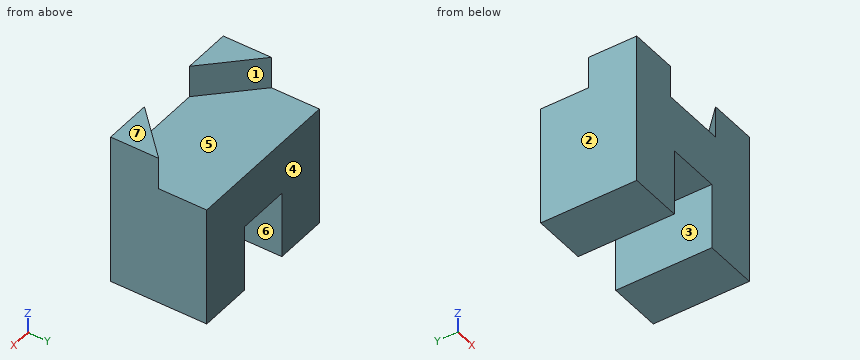
from build123d import *

# Parameters (mm, degrees)
F0_W     = 600
F0_H     = 360
F1_DEPTH = 450
F2_W     = 200
F2_H     = 250
F3_DEPTH = 360.001
F5_DEPTH = 120


with BuildPart() as f1:
    # F0 (on Top) → F1 (new body)
    with BuildSketch(Plane.XY):
        Rectangle(F0_W, F0_H)
    extrude(amount=F1_DEPTH)

    # F2 (on face) → F3 (cut, through all)
    with BuildSketch(Plane.XZ.offset(180)):
        with Locations((0, 125)):
            Rectangle(F2_W, F2_H)
    extrude(amount=-F3_DEPTH, mode=Mode.SUBTRACT)

    # F4 (on face) → F5 (join)
    with BuildSketch(Plane.XY.offset(450)):
        Polygon((-300, 0), (-300, -180), (-120, -180), align=None)
        Polygon((300, 0), (120, -180), (300, -180), align=None)
    extrude(amount=F5_DEPTH)


solid = f1.part
The listing builds one solid part. Answer for the finished solid, in the listing's coordinates (mm). Face numbers are marked on the shaded views. A direction names the side the tool comes from. Coordinates: 2 decimals unless noted, no trailing zeros. Loops run counter-clockwise (first coordinate to the right, second up) from the corner with the lowest first, then second, coordinate; pieces in that order, holes last. Notation, with made-up numbers: M 74,7 L 97,7 A33 cw 97,40 Z; hole C 66.25,4 d2. An arc over 180 degrees is marked long. Answer in a Markdown table with one row per item.
1) Find section C-C (x = -189). Determine the outline of the cut face in (y, z), then the cut area to 3 significant figures.
Answers below:
| item | result |
|---|---|
| outline | M -180,0 L 180,0 L 180,450 L -111,450 L -111,570 L -180,570 Z |
| area | 170,000 mm^2 |
2) Given pin 1 (4 mm diameter, centred on x = 25, y = -51, fed in from +Z), flat-ended and moving along its own axis, determine where the tip first touches the part or whether it passes through.
Answers below:
| item | result |
|---|---|
| pin 1 | z = 450 |
3) Determine the mould class of the marked faces 1, 2, 3 and 4 for opening direction X: released by +X, released by -X, zero draft, split by the parting line, or undercut.
Answers below:
| item | result |
|---|---|
| face 1 | undercut |
| face 2 | released by -X |
| face 3 | undercut |
| face 4 | zero draft |
4) Find section A-A (z = 156). Determine the outline of the cut face in (x, y).
Answers below:
| item | result |
|---|---|
| outline | M -300,-180 L -100,-180 L -100,180 L -300,180 Z; M 100,-180 L 300,-180 L 300,180 L 100,180 Z |
5) Which of the six approach directions +Z, -Z, +X, -X, +Y, -Y give full straight-line access (tool end or side, diameter ignored) to the marked faces 5, 6 and 7?
Answers below:
| item | result |
|---|---|
| face 5 | +Z, +Y |
| face 6 | -Z, +Y, -Y |
| face 7 | +Z, +X, -X, +Y, -Y |
6) Find section D-D (z = 467.5). Determine the outline of the cut face in (x, y), then the cut area to 3 significant figures.
Answers below:
| item | result |
|---|---|
| outline | M -300,-180 L -120,-180 L -300,0 Z; M 120,-180 L 300,-180 L 300,0 Z |
| area | 32,400 mm^2 |
7) Find the intervals of material crossed by probe 1 along X at (y, z) = (145, 147.5); probe 2 along Z at (x, y) = (-192.5, 8.5); probe 3 along Z at (x, y) = (-46, -124), in increasing order.
Answers below:
| item | result |
|---|---|
| probe 1 | -300 to -100, 100 to 300 |
| probe 2 | 0 to 450 |
| probe 3 | 250 to 450 |
8) Find section B-B (y = -145). Determine the outline of the cut face in (x, z).
Answers below:
| item | result |
|---|---|
| outline | M -300,0 L -100,0 L -100,250 L 100,250 L 100,0 L 300,0 L 300,570 L 155,570 L 155,450 L -155,450 L -155,570 L -300,570 Z |
